```python
from build123d import *

# Parameters (mm, degrees)
SKETCH1_R           = 70
BOSS_EXTRUDE1_DEPTH = 18
SKETCH2_R           = 30
CUT_EXTRUDE1_DEPTH  = 101.618089825
SKETCH3_R           = 6.852756537
CUT_EXTRUDE2_DEPTH  = 12.299092
CIRPATTERN1_START   = 5.700908051
CIRPATTERN1_DEPTH   = 12.299091949


# Read off the part's stored shape, not the designer's step: CirPattern1
with BuildPart() as part:
    # Sketch1 → Boss-Extrude1 (new body)
    with BuildSketch(Plane(origin=(0, 0, 0), x_dir=(1, 0, 0), z_dir=(0, 1, 0))):
        with Locations(Location((0, 0, 0), (0, 0, 270))):
            Circle(SKETCH1_R)
    extrude(amount=BOSS_EXTRUDE1_DEPTH)

    # Sketch2 → Cut-Extrude1 (cut, through all)
    with BuildSketch(Plane(origin=(0, 0, 0), x_dir=(1, 0, 0), z_dir=(0, 1, 0))):
        with Locations(Location((0, 0, 0), (0, 0, 270))):
            Circle(SKETCH2_R)
    extrude(amount=CUT_EXTRUDE1_DEPTH, mode=Mode.SUBTRACT)

    # Sketch3 → Cut-Extrude2 (cut)
    with BuildSketch(Plane(origin=(0, 18, 0), x_dir=(1, 0, 0), z_dir=(0, 1, 0))):
        with Locations((-29.836323448, 0)):
            Circle(SKETCH3_R)
    extrude(amount=-CUT_EXTRUDE2_DEPTH, mode=Mode.SUBTRACT)

    # CirPattern1 outline → CirPattern1 (cut)
    with BuildSketch(Plane(origin=(0, 0, 0), x_dir=(1, 0, 0), z_dir=(0, 1, 0)).offset(CIRPATTERN1_START)):
        with BuildLine():
            ThreePointArc((-2.537079389, -29.892527966), (-9.270509831, -28.531695489), (-15.51784675, -25.674820978))
            ThreePointArc((-15.51784675, -25.674820978), (-11.337549223, -34.893388597), (-2.537079389, -29.892527966))
        make_face()
        with BuildLine():
            ThreePointArc((-2.537079389, 29.892527966), (-11.337549223, 34.893388597), (-15.51784675, 25.674820978))
            ThreePointArc((-15.51784675, 25.674820978), (-9.270509831, 28.531695489), (-2.537079389, 29.892527966))
        make_face()
        with BuildLine():
            ThreePointArc((27.645482863, -11.650205032), (24.270509831, -17.633557569), (19.622927434, -22.69230528))
            ThreePointArc((19.622927434, -22.69230528), (29.682089216, -21.565300135), (27.645482863, -11.650205032))
        make_face()
        with BuildLine():
            ThreePointArc((27.645482863, 11.650205032), (29.682089216, 21.565300135), (19.622927434, 22.69230528))
            ThreePointArc((19.622927434, 22.69230528), (24.270509831, 17.633557569), (27.645482863, 11.650205032))
        make_face()
    extrude(amount=CIRPATTERN1_DEPTH, mode=Mode.SUBTRACT)


solid = part.part
```
Geometry check sheet. Reference: the model listing, model coordinates, mm. A direction names the side the tool comes from. Coordinates: 2 decimals unless noted, no trailing zeros. Order: outer loops, then holes, each group sorted by start corner. A loop starts at its lowest first (then second) coordinate and runs counter-clockwise, first axis right, second up. Notation, with made-up numbers: (-10, -32) - (44, -32) arc R22 cw to (44, -23) - close; hole circle Ø10 at (65.25, -19.5). An arc over 180 degrees is marked (long way). Answer in a Markdown table with one row per item. Add a question column.
1. Section check C-C (y = 15.25). Enter the section's corners in (x, z).
2. Draft check along X on faces 1 (the face through (-11, 5.701, -31)), 2 (the face through (32, 18, -1)), 3 (the face through (-18, 7, -24)), 4 (the face through (-42.594, 8.874, -55.55)). Enter one of: +X half, -X half, draft (parallel to the pull), parting line (faces both ways), or undercut.
3. Gauge pin test, flat ends, axial feed: pin 1 Ø2 at (y, z) = (7, -8) entering from -X; pin 2 Ø3 at (y, z) = (5.5, 21) entering from +X; pin 3 Ø8 at (y, z) = (3, -25.5) entering from -X. Record the tip position at first contact, or that the pin passes through.
4. Material ranges on L1, parallel to X at y = 10.25, z = 0; L2, parallel to X at y = 16, z = 26; L3, parallel to Z at x = 4, y = 3, recorded low to high. Write a range as [from, to].
5. Section check B-B (x = 0). Enter the section's corners in (y, z), plus the area to 3 significant figures.
6. Section check D-D (z = 32). Enter the section's corners in (x, y).
7. Access from +Z, -Z, +X, -X, +Y, -Y to the whole of each face (thin tool, end or side, straight path). Record for faces 5 (the face through (-15, 0, 30)), 6 (the face through (-11.19, 11.76, -34.94)).
8. Section check A-A (z = 0). Enter the section's corners in (x, y).
Data:
| question | item | result |
|---|---|---|
| 1 | outline | circle Ø140 at (0, 0); hole (-29.21, -6.82) arc R30 ccw to (-15.52, -25.67) arc R6.85 ccw (long way) to (-2.54, -29.89) arc R30 ccw to (19.62, -22.69) arc R6.85 ccw (long way) to (27.65, -11.65) arc R30 ccw to (27.65, 11.65) arc R6.85 ccw (long way) to (19.62, 22.69) arc R30 ccw to (-2.54, 29.89) arc R6.85 ccw (long way) to (-15.52, 25.67) arc R30 ccw to (-29.21, 6.82) arc R6.85 ccw (long way) to start |
| 2 | face 1 | undercut |
| 2 | face 2 | draft |
| 2 | face 3 | undercut |
| 2 | face 4 | parting line |
| 3 | pin 1 | stops at x = -69.65 |
| 3 | pin 2 | stops at x = 67.23 |
| 3 | pin 3 | stops at x = -66.62 |
| 4 | L1 | x = [-70, -36.69], [30, 70] |
| 4 | L2 | x = [-64.99, -15.65], [14.97, 64.99] |
| 4 | L3 | z = [-69.89, -29.73], [29.73, 69.89] |
| 5 | outline | (0, -70) - (18, -70) - (18, -30) - (0, -30) - close; (0, 30) - (18, 30) - (18, 70) - (0, 70) - close |
| 5 | area | 1,440 mm² |
| 6 | outline | (-62.26, 0) - (62.26, 0) - (62.26, 18) - (-3.4, 18) - (-3.4, 5.7) - (-15.04, 5.7) - (-15.04, 18) - (-62.26, 18) - close |
| 7 | face 5 | +Z, -Z, +X, -X, -Y |
| 7 | face 6 | +Y |
| 8 | outline | (-70, 0) - (-30, 0) - (-30, 5.7) - (-36.69, 5.7) - (-36.69, 18) - (-70, 18) - close; (30, 0) - (70, 0) - (70, 18) - (30, 18) - close |
